```python
from build123d import *

# Parameters (mm, degrees)
SKETCH1_W           = 46.355
SKETCH1_H           = 30.607
SKETCH1_R           = 1.27
BOSS_EXTRUDE1_DEPTH = 1.6764
SKETCH2_W           = 13.97
SKETCH2_H           = 14.224
BOSS_EXTRUDE2_DEPTH = 7.112
SKETCH3_W           = 5.715
SKETCH3_H           = 8.001
BOSS_EXTRUDE3_DEPTH = 2.54
FILLET1_R           = 2.54


with BuildPart() as part:
    # Sketch1 → Boss-Extrude1 (new body)
    with BuildSketch(Plane(origin=(0, 0, 0), x_dir=(1, 0, 0), z_dir=(0, 1, 0))):
        with Locations((23.1775, 15.3035)):
            Rectangle(SKETCH1_W, SKETCH1_H)
        with Locations((4.1275, 26.7335)):
            Circle(SKETCH1_R, mode=Mode.SUBTRACT)
        with Locations((42.2275, 26.7335)):
            Circle(SKETCH1_R, mode=Mode.SUBTRACT)
        with Locations((4.1275, 3.8735)):
            Circle(SKETCH1_R, mode=Mode.SUBTRACT)
        with Locations((42.2275, 3.8735)):
            Circle(SKETCH1_R, mode=Mode.SUBTRACT)
    extrude(amount=BOSS_EXTRUDE1_DEPTH)

    # Sketch2 → Boss-Extrude2 (add)
    with BuildSketch(Plane(origin=(0, 1.6764, 0), x_dir=(1, 0, 0), z_dir=(0, 1, 0))):
        with Locations((45.974, 15.3035)):
            Rectangle(SKETCH2_W, SKETCH2_H)
    extrude(amount=BOSS_EXTRUDE2_DEPTH)

    # Sketch3 → Boss-Extrude3 (add)
    with BuildSketch(Plane(origin=(0, 1.6764, 0), x_dir=(1, 0, 0), z_dir=(0, 1, 0))):
        with Locations((2.8575, 15.3035)):
            Rectangle(SKETCH3_W, SKETCH3_H)
    extrude(amount=BOSS_EXTRUDE3_DEPTH)

    # Fillet1
    fillet1_edges = [part.edges().sort_by_distance(p)[0] for p in [
        (0, 0.8382, -30.607),
        (46.355, 0.8382, -30.607),
        (46.355, 0.8382, 0),
        (0, 0.8382, 0),
    ]]
    fillet(fillet1_edges, radius=FILLET1_R)


solid = part.part
```
Source: CAD feature listing. Evaluate the final solid. Frame: model axes, mm. A direction names the side the tool comes from. Round coordinates to 2 decimals unless told otherwise and drop trailing zeros. Loops run counter-clockwise (first coordinate to the right, second up) from the corner with the lowest first, then second, coordinate; pieces in that order, holes last.
(1) Section query C-C (x = 24.5). Output: boundary loops of the cut face in (y, z).
From the geometry:
outline: (0, -30.61) - (1.68, -30.61) - (1.68, 0) - (0, 0) - close
(2) Section query B-B (z = -10.5). Output: boundary loops of the cut face in (x, y) (3 decimals), and give its area (3 significant figures).
From the geometry:
outline: (0, 0) - (46.355, 0) - (46.355, 1.676) - (52.959, 1.676) - (52.959, 8.788) - (38.989, 8.788) - (38.989, 1.676) - (0, 1.676) - close
area: 177 mm2
(3) Section query A-A (y = 3.5). Output: boundary loops of the cut face in (x, z) (1 decimal), and give its area (3 significant figures).
From the geometry:
outline: (0, -19.3) - (5.7, -19.3) - (5.7, -11.3) - (0, -11.3) - close; (39, -22.4) - (53, -22.4) - (53, -8.2) - (39, -8.2) - close
area: 244 mm2
(4) Contact query for flat-ended pins moving along their axis: pin 1 Ø2 at (x, y) = (49, 6.5) entering from -Z; pin 2 Ø3 at (x, z) = (4.13, -3.87) entering from +Y; pin 3 Ø1.7 at (x, z) = (3, -16) entering from +Y. Output: stop coordinate, or through.
From the geometry:
pin 1: stops at z = -22.42
pin 2: stops at y = 1.68
pin 3: stops at y = 4.22
(5) Access query for faces 4 (the flat face through (5.715, 3, -15)), 5 (the flat face through (46, 5, -8.192)), 6 (the flat face through (50, 1.676, -15)), 7 (the flat face through (3, 4.216, -15)). Directions: +Z, -Z, +X, -X, +Y, -Y. A direction counts if a zero-diameter tool reaches every point of the face in a straight line with its end or side. Return the directions, or none.
From the geometry:
face 4: +Z, -Z, +Y
face 5: +Z, +X, -X, +Y
face 6: +Z, -Z, +X, -Y
face 7: +Z, -Z, -X, +Y
(6) Section query D-D (z = -18). Output: boundary loops of the cut face in (x, y) (3 decimals).
From the geometry:
outline: (0, 0) - (46.355, 0) - (46.355, 1.676) - (52.959, 1.676) - (52.959, 8.788) - (38.989, 8.788) - (38.989, 1.676) - (5.715, 1.676) - (5.715, 4.216) - (0, 4.216) - close
(7) Pull-direction query (Z, two-part tool) for faces 1 (the flat face through (38.989, 5, -15)), 2 (the cylindrical face through (3.12, 0.83, -3.1)), 3 (the flat face through (23, 1, -30.607)); classes: +Z half, -Z half, draft (parallel to the pull), parting line (faces both ways), or undercut.
From the geometry:
face 1: draft
face 2: undercut
face 3: -Z half
(8) Material intervals for probe 1 along Z at (x, y) = (44, 8); probe 2 along X at (y, z) = (1.25, -10.5) (3 decimals); probe 3 along X at (y, z) = (5.75, -13), sorted ascending.
From the geometry:
probe 1: z = -22.42 to -8.19
probe 2: x = 0 to 46.355
probe 3: x = 38.99 to 52.96
